Design review of the part built by this model. Coordinates are the model's own, in mm. A direction names the side the tool comes from. Coordinates: 2 decimals unless noted, no trailing zeros. Answer as a JSON object with one key per item and string values.
```python
from build123d import *

# Parameters (mm, degrees)
SKETCH1_W           = 187.3
SKETCH1_H           = 187.3
BOSS_EXTRUDE1_DEPTH = 6.35
CUT_EXTRUDE2_DEPTH  = 7.35


with BuildPart() as part:
    # Sketch1 → Boss-Extrude1 (new body)
    with BuildSketch(Plane(origin=(0, 0, 0), x_dir=(0, 0, -1), z_dir=(1, 0, 0))):
        Rectangle(SKETCH1_W, SKETCH1_H)
    extrude(amount=BOSS_EXTRUDE1_DEPTH)

    # Sketch3 → Cut-Extrude2 (cut, through all)
    with BuildSketch(Plane(origin=(6.35, 0, 0), x_dir=(0, 0, -1), z_dir=(1, 0, 0))):
        Polygon((-93.65, 66.5), (-89.65, 66.5), (-89.65, 67.71), (-87.3, 67.71), (-87.3, 66.5), (-85.3, 66.5), (-85.3, 63.5), (-87.3, 63.5), (-87.3, 62.29), (-89.65, 62.29), (-89.65, 63.5), (-93.65, 63.5), align=None)
        Polygon((-87.3, -63.5), (-87.3, -62.29), (-89.65, -62.29), (-89.65, -63.5), (-93.65, -63.5), (-93.65, -66.5), (-89.65, -66.5), (-89.65, -67.71), (-87.3, -67.71), (-87.3, -66.5), (-85.3, -66.5), (-85.3, -63.5), align=None)
        Polygon((93.65, -66.5), (89.65, -66.5), (89.65, -67.71), (87.3, -67.71), (87.3, -66.5), (85.3, -66.5), (85.3, -63.5), (87.3, -63.5), (87.3, -62.29), (89.65, -62.29), (89.65, -63.5), (93.65, -63.5), align=None)
        Polygon((87.3, 63.5), (87.3, 62.29), (89.65, 62.29), (89.65, 63.5), (93.65, 63.5), (93.65, 66.5), (89.65, 66.5), (89.65, 67.71), (87.3, 67.71), (87.3, 66.5), (85.3, 66.5), (85.3, 63.5), align=None)
        Polygon((-1.5, 93.65), (-1.5, 89.65), (-2.71, 89.65), (-2.71, 87.3), (-1.5, 87.3), (-1.5, 85.3), (1.5, 85.3), (1.5, 87.3), (2.71, 87.3), (2.71, 89.65), (1.5, 89.65), (1.5, 93.65), align=None)
        Polygon((-2.71, -87.3), (-1.5, -87.3), (-1.5, -85.3), (1.5, -85.3), (1.5, -87.3), (2.71, -87.3), (2.71, -89.65), (1.5, -89.65), (1.5, -93.65), (-1.5, -93.65), (-1.5, -89.65), (-2.71, -89.65), align=None)
    extrude(amount=-CUT_EXTRUDE2_DEPTH, mode=Mode.SUBTRACT)


solid = part.part
```
1) The part is to be moulded in two halves that separate along Y. For faces 1 (the flat face through (3, -66.5, 92)), 2 (the flat face through (3, 63.5, -92)), 3 (the flat face through (3, -1, -93.65)), 4 (the flat face through (3, -93.65, 48)), say which applies: pulls with the +Y half, pulls with the -Y half, needs draft (parallel to the pull), parting line crosses it, or undercut.
Completed:
{"face 1": "undercut", "face 2": "undercut", "face 3": "needs draft", "face 4": "pulls with the -Y half"}
2) For faces 5 (the flat face through (3, 66.5, 92)), 6 (the flat face through (3, -80, -93.65)), 7 (the flat face through (3, -63.5, -92)), 8 (the flat face through (3, 92, 1.5)), 9 (the flat face through (3, 93.65, 48)), list the 3-axis set-ups (+Z, -Z, +X, -X, +Y, -Y) from which the entire face can be reached by the end or side of a thin tool; tool diameter is ignored.
Completed:
{"face 5": "+Z, +X, -X", "face 6": "-Z, +X, -X, +Y, -Y", "face 7": "-Z, +X, -X", "face 8": "+X, -X, +Y", "face 9": "+Z, -Z, +X, -X, +Y"}
3) Wall thickness on probe 1 along Z at (x, y) = (3, -67.5); probe 2 along Z at (x, y) = (2, 65.5): over which ranges is each line inside the solid? List them lowest first.
Completed:
{"probe 1": "-93.65 to -89.65, -87.3 to 87.3, 89.65 to 93.65", "probe 2": "-85.3 to 85.3"}
